Can you work these out from the drawing? Everything is in mm from the part's minimum corner. A direction names the side the tool comes from. Round coordinates to 2 decimals unless told otherwise and drop trailing zeros. Write each loop counter-clockwise with the first axis right and the second up, starting at its lowest first coordinate (ties: lowest second). Pieces come first, ordered by that corner, then holes. Notation, with made-up numbers: (43, -6) - (100, -6) arc R38 ccw to (100, 33) - close; hole circle Ø7 at (-20, 63.25). An arc over 180 degrees is marked (long way). One line per item, written item: value. Start each with the question number.
Item 1: Imagine slicing it at B-B, the plane y = 33.5. Please give me the cut outline in (x, z), then the cut area to 3 significant figures.
Item 2: For P1, Ø2, axis at y = 11, z = 51.5, coming from the +X side; P2, Ø12, axis at x = 65.5, y = 25.5, coming from the +Z side; P3, Ø1.5, axis at x = 88, z = 18, coming from the -Y side (3 decimals), each with a flat end and sliding along its axis, tell me the tip position at first contact or that it passes through.
Item 3: If I drill on line 1 (X direction, y = 36.5, z = 74); line 2 (Y direction, x = 95.5, z = 29.5) (1 decimal), over which ranges is the centre line in solid material (lowest first)?
Item 4: For the marked faces 1, 2, 3 and 4, which set-ups out of +Z, -Z, +X, -X, +Y, -Y let a thin tool reach every point of the face, with its end or its side?
Item 5: Imagine slicing it at C-C, the plane x = 26. Please give me the cut outline in (y, z), then the cut area to 3 significant figures.
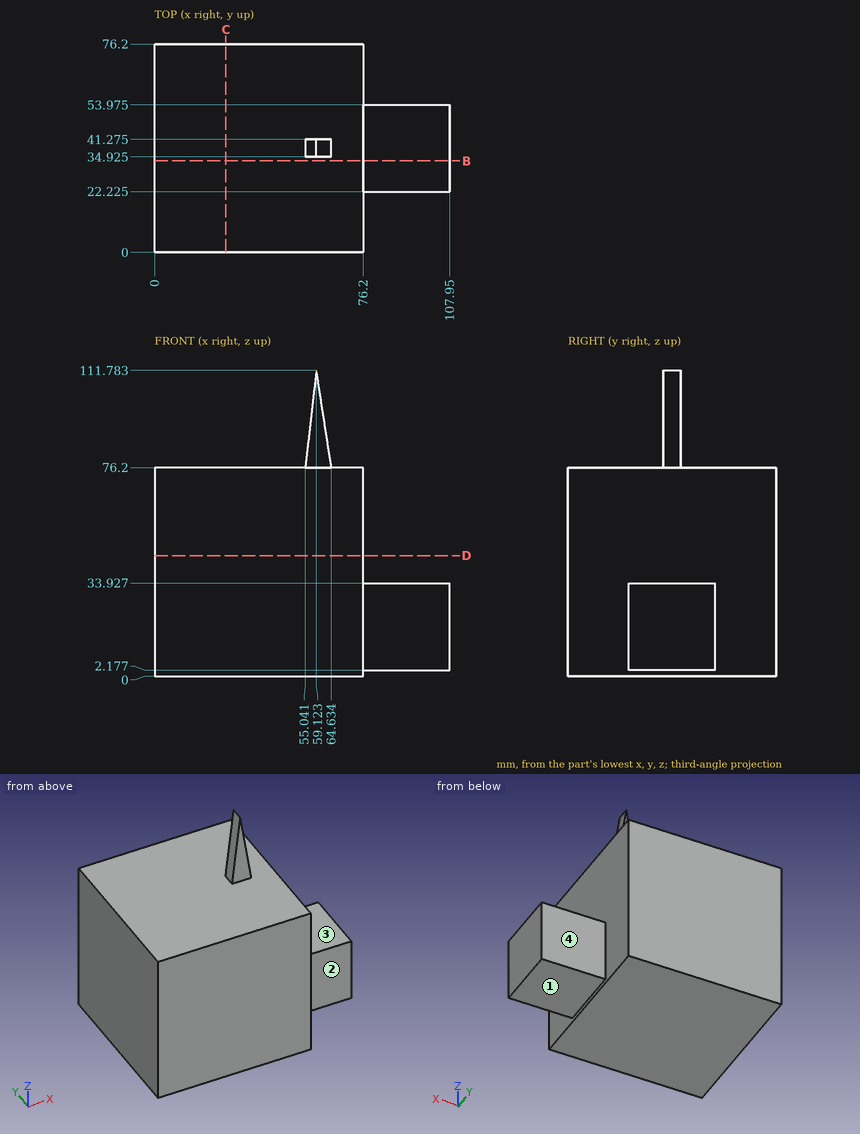
Values follow:
1. outline: (0, 0) - (76.2, 0) - (76.2, 2.18) - (107.95, 2.18) - (107.95, 33.93) - (76.2, 33.93) - (76.2, 76.2) - (0, 76.2) - close
1. area: 6,810 mm^2
2. P1: stops at x = 76.2
2. P2: stops at z = 76.2
2. P3: stops at y = 22.225
3. line 1: x = 0 to 76.2
3. line 2: y = 22.2 to 54
4. face 1: -Z, +X, +Y, -Y
4. face 2: +Z, -Z, +X, -Y
4. face 3: +Z, +X, +Y, -Y
4. face 4: +Z, -Z, +X, +Y
5. outline: (0, 0) - (76.2, 0) - (76.2, 76.2) - (0, 76.2) - close
5. area: 5,810 mm^2
